CAD build for the part. Positions are in the model's coordinates, mm. Coordinates: 2 decimals unless noted, no trailing zeros. Order: outer loops, then holes, each group sorted by start corner. A loop starts at its lowest first (then second) coordinate and runs counter-clockwise, first axis right, second up.
Autodesk Inventor part; units mm, degrees
ref_plane "YZ Plane" through (0, 0, 0) normal (1, 0, 0) x (0, 1, 0)
ref_plane "XZ Plane" through (0, 0, 0) normal (0, 1, 0) x (-1, 0, 0)
ref_plane "XY Plane" through (0, 0, 0) normal (0, 0, 1) x (1, 0, 0)
sketch "Sketch1" plane through (0, 0, 0) normal (0, 1, 0) x (-1, 0, 0)
  line L0 (0, 0) -> (0, 25.4)
  line L1 (0, 0) -> (-279.4, 0)
  line L2 (-279.4, 0) -> (-279.4, 63.5)
  line L3 (0, 25.4) -> (-279.4, 63.5)
  dimension "d0" = 279.4
  dimension "d1" = 25.4
  dimension "d2" = 63.5
extrude "Extrusion1" add sketch "Sketch1" along normal blind 5.9995
sketch "Sketch2" plane through (279.4, 0, 0) normal (0, 0, -1) x (-1, 0, 0)
  line L0 (0, 0) -> (0, 5.9995)
  line L1 (279.4, 0) -> (279.4, 5.9995)
  line L2 (0, 0) -> (279.4, 0)
  point P0 (12.7, 2.9997)
  point P1 (76.2, 2.9997)
  point P2 (139.7, 2.9997)
  point P3 (203.2, 2.9997)
  point P4 (266.7, 2.9997)
  dimension "d5" = 12.7
  dimension "d6" = 12.7
  dimension "d7" = 2.9997
  dimension "d8" = 63.5
  dimension "d9" = 63.5
  dimension "d10" = 63.5
  dimension "d11" = 63.5
hole "Hole1" at (266.7, 2.9997, 0) at (203.2, 2.9997, 0) at (139.7, 2.9997, 0) at (76.2, 2.9997, 0) at (12.7, 2.9997, 0) direction (0, 0, 1) diameter 2.6416 depth 19.05
properties part number "Mount_Support"
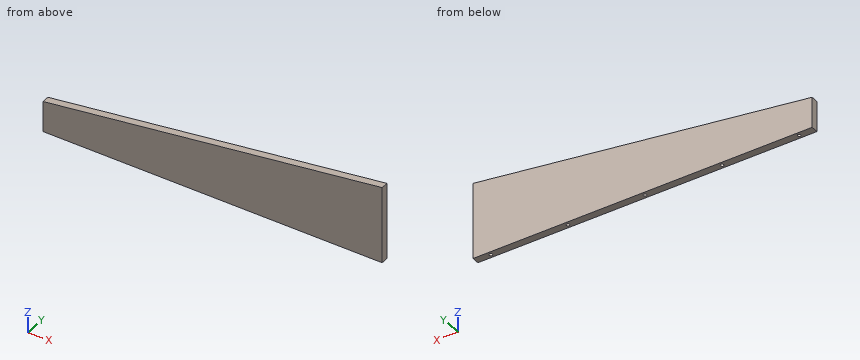
1) Slice it at A-A (z = 11.5). List the corners of the cut face in (x, y).
2) Pin check, flat tips, straight feed: P1, Ø2, axis at x = 203.2, y = 3, coming from the +Z side; P2, Ø0.8, axis at x = 139, y = 3, coming from the -Z side; P3, Ø1.6, axis at x = 266.7, y = 3, coming from the +Z side. Stop position of each tip, or through.
3) Drill centre lines: probe 1 along X at (y, z) = (2.6, 10); probe 2 along Y at (x, z) = (76, 6); probe 3 along X at (y, z) = (1.95, 15.5). Where is each one in solid material? Low to high.
4) Slice it at B-B (x = 214.5). List the corners of the cut face in (y, z), plus the area to 3 significant figures.
5) Slice it at C-C (z = 39). List the corners of the cut face in (x, y).
Worked out:
1. outline: (0, 0) - (279.4, 0) - (279.4, 6) - (0, 6) - close; hole circle Ø2.64 at (12.7, 3); hole circle Ø2.64 at (76.2, 3); hole circle Ø2.64 at (139.7, 3); hole circle Ø2.64 at (203.2, 3); hole circle Ø2.64 at (266.7, 3)
2. P1: stops at z = 53.25
2. P2: stops at z = 19.05
2. P3: stops at z = 61.88
3. probe 1: x = 0 to 11.44, 13.96 to 74.94, 77.46 to 138.44, 140.96 to 201.94, 204.46 to 265.44, 267.96 to 279.4
3. probe 2: y = 0 to 1.69, 4.31 to 6
3. probe 3: x = 0 to 11.9, 13.5 to 75.4, 77 to 138.9, 140.5 to 202.4, 204 to 265.9, 267.5 to 279.4
4. outline: (0, 0) - (6, 0) - (6, 54.65) - (0, 54.65) - close
4. area: 328 mm2
5. outline: (99.73, 0) - (279.4, 0) - (279.4, 6) - (99.73, 6) - close
